Verification items for the finished model (mm, model axes). A direction names the side the tool comes from. Coordinates: 2 decimals unless noted, no trailing zeros. Loops run counter-clockwise (first coordinate to the right, second up) from the corner with the lowest first, then second, coordinate; pieces in that order, holes last. Notation, with made-up numbers: (26.25, -3) -> (85.25, -3) arc R24 cw to (85.25, 36) -> close; hole circle Ø6 at (-22, 40). An arc over 180 degrees is marked (long way). Use CSV: the item, a comma, the result in double quotes. Start each with the question number.
```python
from build123d import *

# Parameters (mm, degrees)
SKETCH2_R                = 26.25
BOSS_EXTRUDE2_DEPTH      = 147.5
BOSS_EXTRUDE4_DEPTH      = 15.416
BOSS_EXTRUDE4_DEPTH_BACK = 45.4
SKETCH3_R                = 26.25


with BuildPart() as part:
    # Sketch2 → Boss-Extrude2 (new body)
    with BuildSketch(Plane.XY):
        with Locations((-32.979772941, 24.734829706)):
            Circle(SKETCH2_R)
    extrude(amount=BOSS_EXTRUDE2_DEPTH)

    # Sketch3 → Boss-Extrude4 (add, two sides: drawn at the far end of the back side and taken through both)
    with BuildSketch(Plane(origin=(0, 0, 0), x_dir=(1, 0, 0), z_dir=(0, 1, 0)).offset(-BOSS_EXTRUDE4_DEPTH_BACK)):
        with Locations(Location((-33.04352384, -26.794047718, 0), (0, 0, 270))):
            Circle(SKETCH3_R)
    extrude(amount=BOSS_EXTRUDE4_DEPTH + BOSS_EXTRUDE4_DEPTH_BACK)


solid = part.part
```
1. Scan lines: line 1 (Y direction, x = -32, z = 115); line 2 (Y direction, x = -49.5, z = 94.5); line 3 (Z direction, x = -20, y = -17.5). Record each from-to range of solid material in increasing order.
2. Cross-section at B-B, the plane y = 11. Record the boundary of the cut face in (x, z), plus the area to 3 significant figures.
3. Cross-section at C-C, the plane z = 38.5. Record the boundary of the cut face in (x, y).
4. Cross-section at D-D, the plane y = 45. Record the boundary of the cut face in (x, z), plus the area to 3 significant figures.
5. Cross-section at A-A, the plane x = -21. Record the boundary of the cut face in (y, z).
6. Set-up check for faces 1 (the cylindrical face through (-56.33, -22.18, 38.91)), 2 (the flat face through (-33, 25, 0)): record each of +Z, -Z, +X, -X, +Y, -Y from which the full face is reachable in a straight line by a thin tool's end or side.
7. Depth check by flat-ended pin: pin 1 (6 mm diameter, centred on y = 40.5, z = 101.5, fed in from -X); pin 2 (3 mm diameter, centred on x = -24, y = -6, fed in from -Z); pin 3 (5 mm diameter, centred on y = 38, z = 93.5, fed in from -X). Enter the tip coordinate at first touch or a pass-through.
Solution:
1,line 1,"y = -1.5 to 50.97"
1,line 2,"y = 4.34 to 45.13"
1,line 3,"z = 4.01 to 49.57"
2,outline,"(-55.35, 0) -> (-10.61, 0) -> (-10.61, 13.16) arc R26.25 ccw to (-10.61, 40.42) -> (-10.61, 147.5) -> (-55.35, 147.5) -> (-55.35, 40.63) arc R26.25 ccw to (-55.35, 12.96) -> close"
2,area,"6,740 mm2"
3,outline,"(-56.54, -45.4) -> (-9.55, -45.4) -> (-9.55, 12.9) arc R26.25 ccw (long way) to (-56.54, 13.16) -> close"
4,outline,"(-49.66, 0) -> (-16.29, 0) -> (-16.29, 147.5) -> (-49.66, 147.5) -> close"
4,area,"4,920 mm2"
5,outline,"(-45.4, 3.47) -> (1.38, 3.47) -> (1.38, 0) -> (48.09, 0) -> (48.09, 147.5) -> (1.38, 147.5) -> (1.38, 50.12) -> (-45.4, 50.12) -> close"
6,face 1,"-Y"
6,face 2,"-Z, +X, -X, +Y, -Y"
7,pin 1,"stops at x = -55.92"
7,pin 2,"stops at z = 1.65"
7,pin 3,"stops at x = -56.92"
